The model under review builds one solid part; all positions refer to its coordinate system, in mm. A direction names the side the tool comes from. Give positions to 0.01 mm unless a question says otherwise; leave off trailing zeros. Order: outer loops, then holes, each group sorted by start corner. A loop starts at its lowest first (then second) coordinate and runs counter-clockwise, first axis right, second up. Notation, with made-up numbers: (19, -8) - (42, -8) arc R28 cw to (42, 11) - close; hole circle Ø3 at (-33, 78). An arc over 180 degrees is marked (long way). Use a Markdown table: item, result. Add a question column.
```python
from build123d import *

# Parameters (mm, degrees)
ESQUISSE1_W             = 100.91
ESQUISSE1_H             = 40.386
BOSS_EXTRU_1_DEPTH      = 101.6
ENL_V_MAT_EXTRU_1_DEPTH = 101.6
ENL_V_MAT_EXTRU_2_DEPTH = 149.783121005
ESQUISSE5_R             = 3.975
ENL_V_MAT_EXTRU_3_DEPTH = 20
ESQUISSE6_R             = 3.937
ENL_V_MAT_EXTRU_4_DEPTH = 20
ESQUISSE7_R             = 3.937
ENL_V_MAT_EXTRU_5_DEPTH = 20
ESQUISSE8_R             = 3.937
ENL_V_MAT_EXTRU_6_DEPTH = 20
ESQUISSE9_R             = 6.35
ENL_V_MAT_EXTRU_7_DEPTH = 149.783121005
ESQUISSE10_R            = 9.525
ENL_V_MAT_EXTRU_8_DEPTH = 7.35
ESQUISSE11_R            = 12.7
ENL_V_MAT_EXTRU_9_DEPTH = 20.65


with BuildPart() as part:
    # Esquisse1 → Boss.-Extru.1 (new body)
    with BuildSketch(Plane.XY):
        with Locations((50.455, 20.193)):
            Rectangle(ESQUISSE1_W, ESQUISSE1_H)
    extrude(amount=BOSS_EXTRU_1_DEPTH)

    # Esquisse3 → Enlèv. mat.-Extru.1 (cut)
    with BuildSketch(Plane(origin=(0, 0, 0), x_dir=(-1, 0, 0), z_dir=(0, 0, -1))):
        Polygon((-100.91, 20.193), (-80.717, 0), (-100.91, 0), align=None)
        Polygon((0, 0), (0, 20.193), (-20.193, 0), align=None)
    extrude(amount=-ENL_V_MAT_EXTRU_1_DEPTH, mode=Mode.SUBTRACT)

    # Esquisse4 → Enlèv. mat.-Extru.2 (cut, through all)
    with BuildSketch(Plane(origin=(0, 0, 0), x_dir=(-1, 0, 0), z_dir=(0, 0, -1))):
        Polygon((-100.91, 20.193), (-80.717, 40.386), (-100.91, 40.386), align=None)
        Polygon((0, 40.386), (0, 20.193), (-20.193, 40.386), align=None)
    extrude(amount=-ENL_V_MAT_EXTRU_2_DEPTH, mode=Mode.SUBTRACT)

    # Esquisse5 → Enlèv. mat.-Extru.3 (cut)
    with BuildSketch(Plane(origin=(60.5515, 60.5515, 0), x_dir=(0, 0, -1), z_dir=(0.7071067811865488, 0.7071067811865464, 0))):
        with Locations(Location((-88.9, -42.796930825, 0), (0, 0, 90))):
            Circle(ESQUISSE5_R)
        with Locations(Location((-12.7, -42.796930825, 0), (0, 0, 90))):
            Circle(ESQUISSE5_R)
    extrude(amount=-ENL_V_MAT_EXTRU_3_DEPTH, mode=Mode.SUBTRACT)

    # Esquisse6 → Enlèv. mat.-Extru.4 (cut)
    with BuildSketch(Plane(origin=(10.0965, 10.0965, 0), x_dir=(0, 0, 1), z_dir=(-0.7071067811865475, -0.7071067811865476, 0))):
        with Locations(Location((12.7, 0, 0), (0, 0, 270))):
            Circle(ESQUISSE6_R)
        with Locations(Location((88.9, 0, 0), (0, 0, 270))):
            Circle(ESQUISSE6_R)
    extrude(amount=-ENL_V_MAT_EXTRU_4_DEPTH, mode=Mode.SUBTRACT)

    # Esquisse7 → Enlèv. mat.-Extru.5 (cut)
    with BuildSketch(Plane(origin=(-10.0965, 10.0965, 0), x_dir=(0, 0, 1), z_dir=(-0.7071067811865488, 0.7071067811865464, 0))):
        with Locations(Location((31.75, 28.557214465, 0), (0, 0, 270))):
            Circle(ESQUISSE7_R)
        with Locations(Location((69.85, 28.557214465, 0), (0, 0, 270))):
            Circle(ESQUISSE7_R)
    extrude(amount=-ENL_V_MAT_EXTRU_5_DEPTH, mode=Mode.SUBTRACT)

    # Esquisse8 → Enlèv. mat.-Extru.6 (cut)
    with BuildSketch(Plane(origin=(40.3585, -40.3585, 0), x_dir=(0, 0, -1), z_dir=(0.7071067811865475, -0.7071067811865476, 0))):
        with Locations(Location((-69.85, 71.35414529, 0), (0, 0, 90))):
            Circle(ESQUISSE8_R)
        with Locations(Location((-31.75, 71.35414529, 0), (0, 0, 90))):
            Circle(ESQUISSE8_R)
    extrude(amount=-ENL_V_MAT_EXTRU_6_DEPTH, mode=Mode.SUBTRACT)

    # Esquisse9 → Enlèv. mat.-Extru.7 (cut, through all)
    with BuildSketch(Plane(origin=(0, 0, 0), x_dir=(-1, 0, 0), z_dir=(0, 0, -1))):
        with Locations((-50.455, 20.193)):
            Circle(ESQUISSE9_R)
    extrude(amount=-ENL_V_MAT_EXTRU_7_DEPTH, mode=Mode.SUBTRACT)

    # Esquisse10 → Enlèv. mat.-Extru.8 (cut)
    with BuildSketch(Plane(origin=(0, 0, 0), x_dir=(-1, 0, 0), z_dir=(0, 0, -1))):
        with Locations((-50.455, 20.193)):
            Circle(ESQUISSE10_R)
    extrude(amount=-ENL_V_MAT_EXTRU_8_DEPTH, mode=Mode.SUBTRACT)

    # Esquisse11 → Enlèv. mat.-Extru.9 (cut)
    with BuildSketch(Plane.XY.offset(101.6)):
        with Locations((50.455, 20.193)):
            Circle(ESQUISSE11_R)
    extrude(amount=-ENL_V_MAT_EXTRU_9_DEPTH, mode=Mode.SUBTRACT)


solid = part.part
```
Q1. We need section A-A (z = 51). Write out the cut boundary in (x, y) (3 decimals).
Q2. We need section C-C (z = 68). Write out the cut boundary in (x, y) (3 decimals), plus the area to 3 significant figures.
Q3. We need section D-D (x = 14.5). Count the separate pieces of the cut face and the enclosed holes in it, plus the area to 3 significant figures.
Q4. Clearance check with flat-ended pins moving along their axes: P1, Ø20.5, axis at x = 50.455, y = 20.193, coming from the +Z side; P2, Ø2, axis at y = 18.5, z = 38.5, coming from the +X side; P3, Ø6, axis at y = 34, z = 79, coming from the +X side. State where each tip first meets the part, or that it passes through.
Q5. Wall thickness on probe 1 along Z at (x, y) = (13, 29); probe 2 along X at (y, z) = (16, 71); probe 3 along X at (y, z) = (21, 70.5): over which ranges is each line inside the solid? List them lowest first.
Q6. We need section B-B (x = 52). Write out the cut boundary in (y, z).
Q7. Draft analysis for pull direction X (two halves, no side actions). For faces 4 (the flat face through (9.955, 10.238, 50.089)), 5 (the flat face through (44.6, 23.2, 80.95)), 6 (the flat face through (50, 0, 50)), state which applies: pulls with the +X half, pulls with the -X half, needs draft (parallel to the pull), parting line crosses it, or undercut.
Q8. Machinability: for faces 1 (the flat face through (90.955, 30.148, 50.089)), 2 (the flat face through (76.71, 16.11, 88.96)), 3 (the cylindrical face through (62.569, 24.008, 91.42)), which of the approach directions +Z, -Z, +X, -X, +Y, -Y give a long, thin tool a straight path to every point of the face, cutting with its end or side? Answer none if there is none.
Here are the results:
| question | item | result |
|---|---|---|
| 1 | outline | (0, 20.193) - (20.193, 0) - (80.717, 0) - (100.91, 20.193) - (80.717, 40.386) - (20.193, 40.386) - close; hole circle Ø12.7 at (50.455, 20.193) |
| 2 | outline | (0, 20.193) - (20.193, 0) - (80.717, 0) - (88.356, 7.639) - (74.214, 21.781) - (79.129, 26.696) - (93.271, 12.554) - (100.91, 20.193) - (80.717, 40.386) - (20.193, 40.386) - (12.554, 32.747) - (26.696, 18.605) - (21.781, 13.69) - (7.639, 27.832) - close; hole circle Ø12.7 at (50.455, 20.193) |
| 2 | area | 2,860 mm2 |
| 3 | separate pieces | 1 |
| 3 | enclosed holes | 4 |
| 3 | area | 2,670 mm2 |
| 4 | P1 | z = 80.95 |
| 4 | P2 | x = 100.22 |
| 4 | P3 | x = 90.1 |
| 5 | probe 1 | 0 to 27.98, 35.52 to 66.08, 73.62 to 101.6 |
| 5 | probe 2 | 4.19 to 19.06, 24.09 to 45.69, 55.22 to 79.59, 90.23 to 96.72 |
| 5 | probe 3 | 0.81 to 13.89, 24.88 to 44.16, 56.75 to 74.42, 85.4 to 100.1 |
| 6 | outline | (0, 0) - (10.79, 0) - (10.79, 7.35) - (14.03, 7.35) - (14.03, 80.95) - (7.59, 80.95) - (7.59, 101.6) - (0, 101.6) - close; (26.35, 7.35) - (29.59, 7.35) - (29.59, 0) - (40.39, 0) - (40.39, 101.6) - (32.8, 101.6) - (32.8, 80.95) - (26.35, 80.95) - close |
| 7 | face 4 | pulls with the -X half |
| 7 | face 5 | undercut |
| 7 | face 6 | needs draft |
| 8 | face 1 | +Z, -Z, +X, +Y |
| 8 | face 2 | none |
| 8 | face 3 | +Z |
